Input: dimensioned drawing with shaded views. Units: mm. Origin: part minimum x, y, z. A direction names the side the tool comes from. Coordinates: 2 decimals unless noted, no trailing zeros. Order: outer loops, then holes, each group sorted by start corner. A loop starts at its lowest first (then second) coordinate and runs counter-clockwise, first axis right, second up. Notation, with made-up numbers: (11.25, 29.5) - (30.25, 29.5) arc R18 cw to (30.25, 56.5) - close; hole circle Ø3 at (87.5, 18.25). An arc over 180 degrees is marked (long way). One line per question, with ' | ' between items. Start each with the question number.
(1) Contact query for flat-ended pins moving along their axis: P1, Ø15, axis at x = 22, y = 20.5, coming from the +Z side; P2, Ø10, axis at x = 37.5, z = 57, coming from the +Y side. Output: stop coordinate, or through.
(2) Section C-C (x = 7.5). Return the cut outline in (y, z), then the cut area to 3 significant figures.
(3) Section D-D (y = 27.5). Return the cut outline in (x, z).
(4) Section A-A (z = 50). Return the cut outline in (x, y), then the cut area to 3 significant figures.
(5) Line query: line 1 along X through (y, z) = (2.25, 50); line 2 along Z through (x, y) = (30, 19.5); line 3 along Y through (x, z) = (19.5, 23). Output: solid intervals per line, ascending.
(6) Section B-B (x = 14.5). Return the cut outline in (y, z), then the cut area to 3 significant figures.
(7) Draft query along Z for the marked faces 3, 4 and 5. Return one class per face: +Z half, -Z half, draft (parallel to the pull), parting line (faces both ways), or undercut.
(8) Access query for the marked faces 1 and 2. Directions: +Z, -Z, +X, -X, +Y, -Y. A direction counts if a zero-diameter tool reaches every point of the face in a straight line with its end or side. Return the directions, or none.
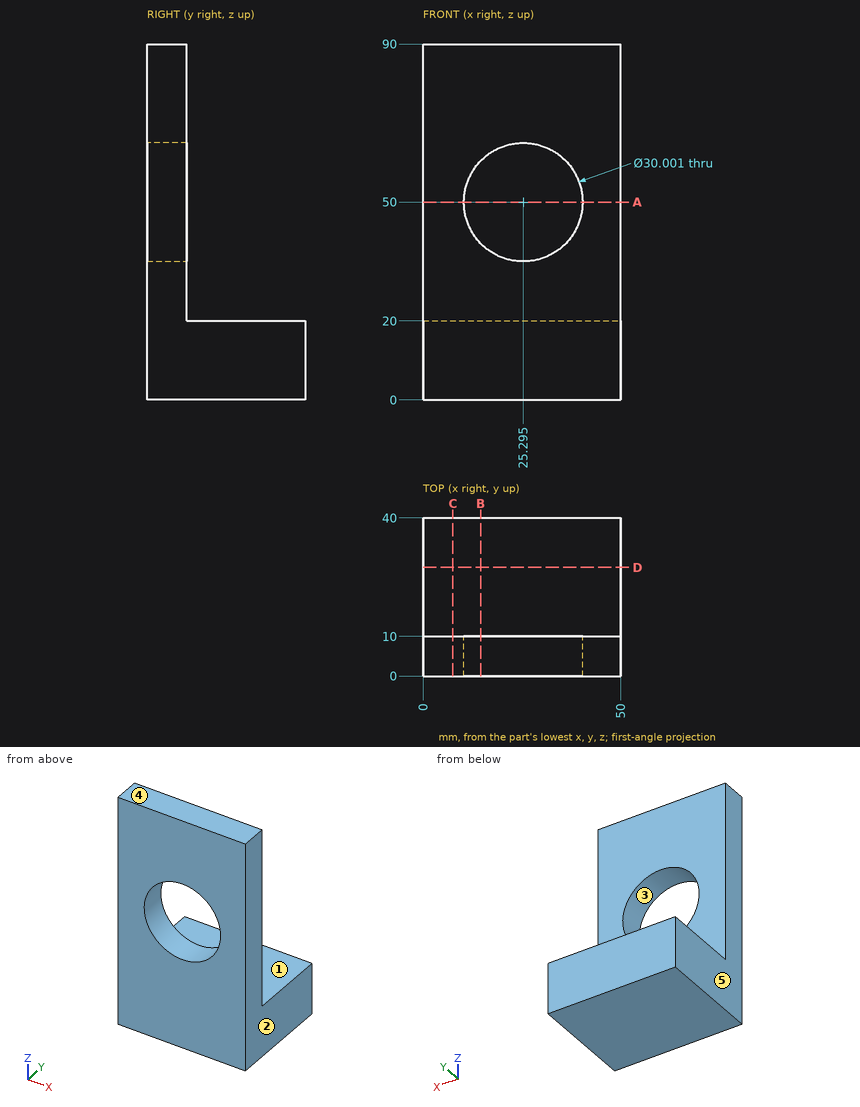
Response values:
1) P1: stops at z = 20 | P2: stops at y = 10
2) outline: (0, 0) - (40, 0) - (40, 20) - (10, 20) - (10, 90) - (0, 90) - close | area: 1,500 mm²
3) outline: (0, 0) - (50, 0) - (50, 20) - (0, 20) - close
4) outline: (0, 0) - (10.29, 0) - (10.29, 10) - (0, 10) - close; (40.3, 0) - (50, 0) - (50, 10) - (40.3, 10) - close | area: 200 mm²
5) line 1: x = 0 to 10.29, 40.3 to 50 | line 2: z = 0 to 20 | line 3: y = 0 to 10
6) outline: (0, 0) - (40, 0) - (40, 20) - (10, 20) - (10, 39.58) - (0, 39.58) - close; (0, 60.42) - (10, 60.42) - (10, 90) - (0, 90) - close | area: 1,290 mm²
7) face 3: undercut | face 4: +Z half | face 5: draft
8) face 1: +Z, +X, -X, +Y | face 2: +Z, -Z, +X, +Y, -Y
